Study the drawing (mm; zero at the part's minimum x, y, z) and answer. A direction names the side the tool comes from. Give positions to 0.01 mm unless a question says otherwise; leave off trailing zeros. Order: outer loops, then holes, each group sorted by start corner. A loop starts at its lowest first (then second) coordinate and runs counter-clockwise, first axis right, second up. Notation, with made-up numbers: (70, 21.25) - (112, 21.25) arc R26 ccw to (112, 46.25) - close; hole circle Ø6 at (73, -39). An arc over 180 degrees is marked (long way). Return JSON: item names as keys, results as strings.
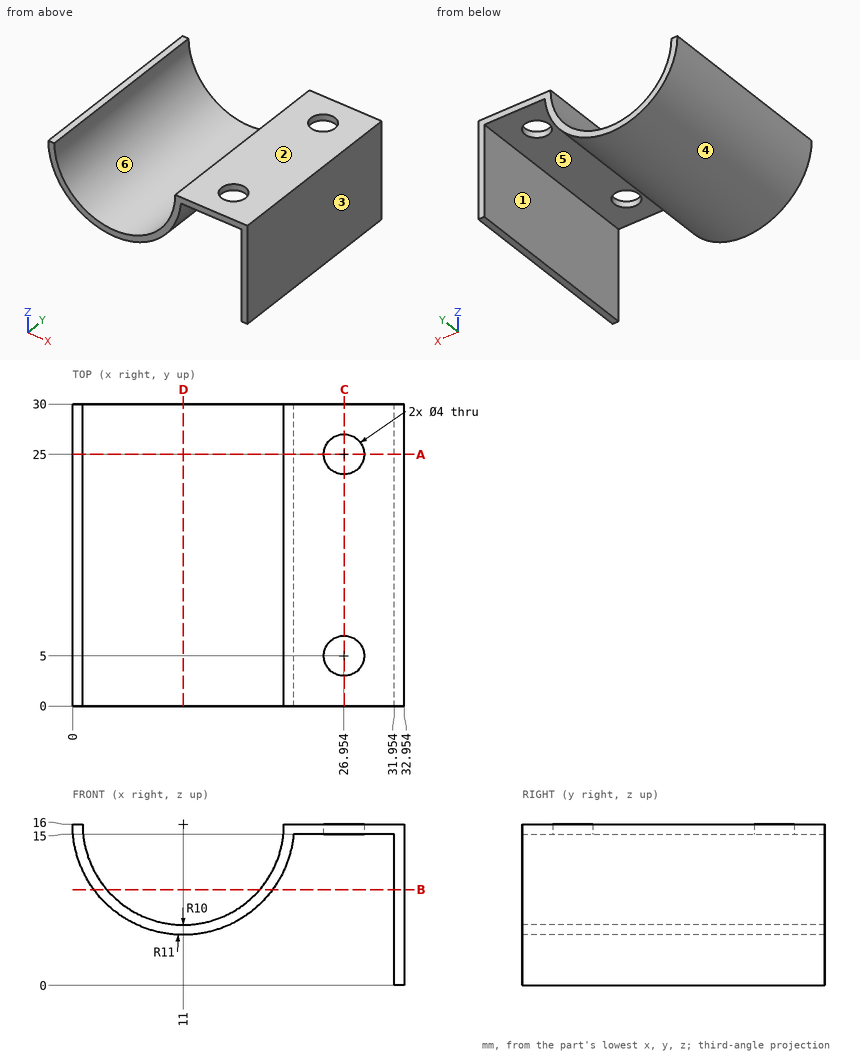
Q1. For the marked faces 5 and 6, determine the directions among +Z, -Z, +X, -X, +Y, -Y from which every point of the face is accessible in a straight line to the end or side of a thin tool.
Values:
{"face 5": "-Z, +Y, -Y", "face 6": "+Z, +Y, -Y"}
Q2. Consider L1, parallel to X at y = 14.5, z = 10 (1 decimal); L2, parallel to X at y = 2, z = 2.5 (1 decimal); L3, parallel to X at y = 16.75, z = 14 (1 decimal). Determine where each line is inside the solid, lowest interval first.
Values:
{"L1": "x = 1.8 to 3, 19 to 20.2, 32 to 33", "L2": "x = 32 to 33", "L3": "x = 0.2 to 1.2, 20.8 to 21.8, 32 to 33"}
Q3. A cutting plane is placed at D-D (x = 11). Write down the section's boundary in (y, z).
Values:
{"outline": "(0, 5) - (30, 5) - (30, 6) - (0, 6) - close"}
Q4. A cutting plane is placed at B-B (z = 9.5). Write down the section's boundary in (x, y) (1 decimal).
Values:
{"outline": "(2.1, 0) - (3.4, 0) - (3.4, 30) - (2.1, 30) - close; (18.6, 0) - (19.9, 0) - (19.9, 30) - (18.6, 30) - close; (32, 0) - (33, 0) - (33, 30) - (32, 30) - close"}
Q5. Given pin 1 (4.5 mm diameter, centred on x = 26.95, y = 25, fed in from -Z); pin 2 (8 mm diameter, centred on y = 23, z = 11.5, fed in from -X); pin 3 (4 mm diameter, centred on y = 10.5, z = 10.5, fed in from -X), each flat-ended and moving along its own axis, determine where each tip first touches the part or whether it passes through.
Values:
{"pin 1": "stops at z = 15", "pin 2": "stops at x = 0.01", "pin 3": "stops at x = 0.57"}
Q6. Determine the mould class of the marked faces 1, 2, 3 and 4 for opening direction X: released by +X, released by -X, zero draft, split by the parting line, or undercut.
Values:
{"face 1": "undercut", "face 2": "zero draft", "face 3": "released by +X", "face 4": "undercut"}
Q7. A cutting plane is placed at A-A (y = 25). Write down the section's boundary in (x, z) (1 decimal).
Values:
{"outline": "(0, 16) arc R11 ccw to (22, 15) - (25, 15) - (25, 16) - (21, 16) arc R10 cw to (1, 16) - close; (29, 15) - (32, 15) - (32, 0) - (33, 0) - (33, 16) - (29, 16) - close"}
Q8. A cutting plane is placed at C-C (x = 27). Write down the section's boundary in (y, z).
Values:
{"outline": "(0, 15) - (3, 15) - (3, 16) - (0, 16) - close; (7, 15) - (23, 15) - (23, 16) - (7, 16) - close; (27, 15) - (30, 15) - (30, 16) - (27, 16) - close"}
